CAD build for the part. Positions are in the model's coordinates, mm. Face numbers are marked on the shaded views. A direction names the side the tool comes from. Coordinates: 2 decimals unless noted, no trailing zeros. Order: outer loops, then holes, each group sorted by start corner. A loop starts at its lowest first (then second) coordinate and runs counter-clockwise, first axis right, second up. Notation, with made-up numbers: (85.5, 88.5) - (90.5, 88.5) arc R21 cw to (90.5, 124.5) - close; hole circle Ø9 at (-24, -0.5). An arc over 180 degrees is marked (long way). Write each question's results on one line, items separated by ' | '. Start each with the question number.
Q1. Wall check: probe 1 along Y at (x, z) = (-3.81, -9.45); probe 2 along Z at (x, y) = (-4.75, 5) (1 decimal); probe 3 along X at (y, z) = (0, 8.8). Give the ranges that are in metal, low to high.
Q2. Which spindle directions (+Z, -Z, +X, -X, +Y, -Y) get a long thin tool onto all of the face, cutting with end or side? Do the marked faces 1 and 2. Say none if no direction does.
Q3. Pull direction Z, two halves, no side cores. Call the marked faces 3, 4, 5 and 6: released by +Z, released by -Z, zero draft, split by the parting line, or undercut.
Q4. Pin check, flat tip, straight feed: P1, Ø1, axis at y = 4, z = -3.5, coming from the -X side. Stop position of the tip, or through.
Q5. Band-saw the part on B-B, the plane y = 0. Count the separate pieces of the cut face and the enclosed holes in it, then the cut area to 3 significant figures.
Q6. Band-saw the part on D-D, the plane z = -7.75. Write the cut outline in (x, y).
Q7. Band-saw the part on A-A, the plane x = -3.81. Write the cut outline in (y, z) (1 decimal).
Q8. Band-saw the part on C-C, the plane x = -8.25. Write the cut outline in (y, z) (1 decimal), then the cut area to 3 significant figures.
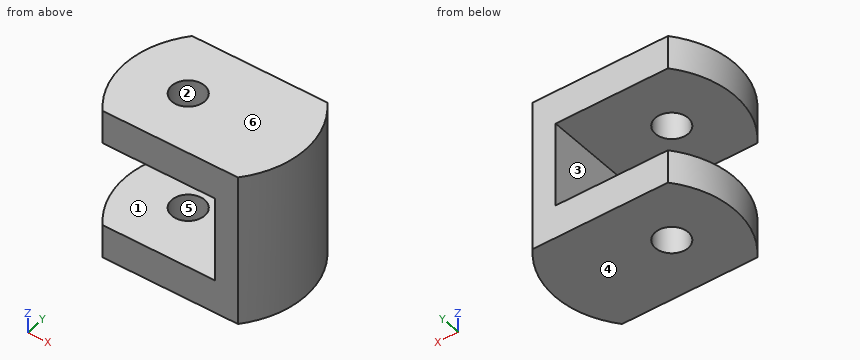
```python
from build123d import *

# Parameters (mm, degrees)
SKETCH1_W               = 12.7
SKETCH1_H               = 21.59
CUT_EXTRUDE1_DEPTH      = 21.955
CUT_EXTRUDE1_DEPTH_BACK = 21.955
SKETCH3_W               = 19.05
SKETCH3_H               = 12.065
CUT_EXTRUDE2_DEPTH      = 21.955
CUT_EXTRUDE2_DEPTH_BACK = 21.955
SKETCH4_W               = 19.231618108
SKETCH4_H               = 5.318049176
CUT_EXTRUDE3_DEPTH      = 27.386441902
CUT_EXTRUDE3_DEPTH_BACK = 27.386441902
SKETCH5_R               = 2.3241


with BuildPart() as part:
    # Sketch1 → Revolve1 (revolve)
    with BuildSketch(Plane(origin=(0, 0, 0), x_dir=(1, 0, 0), z_dir=(0, 1, 0))):
        with Locations((6.35, 0)):
            Rectangle(SKETCH1_W, SKETCH1_H)
    revolve(axis=Axis((0, 0, 10.795), (0, 0, -1)))

    # Sketch3 → Cut-Extrude1 (cut, two sides: drawn at the far end of the back side and taken through both)
    with BuildSketch(Plane(origin=(0, 0, 0), x_dir=(1, 0, 0), z_dir=(0, 1, 0)).offset(-CUT_EXTRUDE1_DEPTH_BACK)):
        with Locations((-3.175, 0)):
            Rectangle(SKETCH3_W, SKETCH3_H)
    extrude(amount=CUT_EXTRUDE1_DEPTH + CUT_EXTRUDE1_DEPTH_BACK, mode=Mode.SUBTRACT)

    # Sketch4 → Cut-Extrude2 (cut, two sides: drawn at the far end of the back side and taken through both)
    with BuildSketch(Plane.XY.offset(-CUT_EXTRUDE2_DEPTH_BACK)):
        Polygon((-9.615809054, 8.296156715), (9.615809054, 8.296156715), (9.615809054, 14.116385036), (-9.615809054, 13.939663028), align=None)
        with Locations((0, -10.955181303)):
            Rectangle(SKETCH4_W, SKETCH4_H)
    extrude(amount=CUT_EXTRUDE2_DEPTH + CUT_EXTRUDE2_DEPTH_BACK, mode=Mode.SUBTRACT)

    # Sketch5 → Cut-Extrude3 (cut, two sides: drawn at the far end of the back side and taken through both)
    with BuildSketch(Plane.XY.offset(10.795).offset(-CUT_EXTRUDE3_DEPTH_BACK)):
        with Locations((-3.81, 0)):
            Circle(SKETCH5_R)
    extrude(amount=CUT_EXTRUDE3_DEPTH + CUT_EXTRUDE3_DEPTH_BACK, mode=Mode.SUBTRACT)


solid = part.part
```
Results below:
1) probe 1: y = -8.3 to -2.32, 2.32 to 8.3 | probe 2: z = -10.8 to -6, 6 to 10.8 | probe 3: x = -12.7 to -6.13, -1.49 to 12.7
2) face 1: -X, +Y, -Y | face 2: +Z, -Z
3) face 3: undercut | face 4: released by -Z | face 5: zero draft | face 6: released by +Z
4) P1: stops at x = 6.35
5) separate pieces: 3 | enclosed holes: 0 | area: 274 mm²
6) outline: (-9.62, -8.3) - (9.62, -8.3) arc R12.7 ccw to (9.62, 8.3) - (-9.62, 8.3) arc R12.7 ccw to start; hole circle Ø4.65 at (-3.81, 0)
7) outline: (-8.3, -10.8) - (-2.3, -10.8) - (-2.3, -6) - (-8.3, -6) - close; (-8.3, 6) - (-2.3, 6) - (-2.3, 10.8) - (-8.3, 10.8) - close; (2.3, -10.8) - (8.3, -10.8) - (8.3, -6) - (2.3, -6) - close; (2.3, 6) - (8.3, 6) - (8.3, 10.8) - (2.3, 10.8) - close
8) outline: (-8.3, -10.8) - (8.3, -10.8) - (8.3, -6) - (-8.3, -6) - close; (-8.3, 6) - (8.3, 6) - (8.3, 10.8) - (-8.3, 10.8) - close | area: 158 mm²
